Input: part model. Units: mm. Frame: model coordinates. Face numbers are marked on the shaded views. A direction names the side the tool comes from. Give positions to 0.01 mm unless a question says otherwise; leave off trailing zeros. Loops run counter-clockwise (first coordinate to the right, second up) from the corner with the lowest first, then second, coordinate; pieces in that order, holes last. Notation, with made-up numbers: (9, 32.25) - (20, 32.25) arc R3 ccw to (20, 36.25) - close; hole circle Ø1 at (7, -25). An arc over 180 degrees is marked (long way). One line per question, with ' | ' between items. Start each with the question number.
from build123d import *

# Parameters (mm, degrees)
SKETCH_1_R          = 25
SKETCH_1_R_2        = 10
EXTRUDE_1_DEPTH     = 50
EXTRUDE_2_DEPTH     = 12.5
CUT_EXTRUDE_1_DEPTH = 74.993242935
SKETCH_5_R          = 5
CUT_EXTRUDE_2_DEPTH = 124.51619327


with BuildPart() as part:
    # 草图1 → 凸台-拉伸1 (new body)
    with BuildSketch(Plane(origin=(0, 0, 0), x_dir=(1, 0, 0), z_dir=(0, 1, 0))):
        with Locations(Location((0, 0, 0), (0, 0, 270))):
            Circle(SKETCH_1_R)
        with Locations(Location((0, 0, 0), (0, 0, 270))):
            Circle(SKETCH_1_R_2, mode=Mode.SUBTRACT)
    extrude(amount=EXTRUDE_1_DEPTH)

    # 草图2 → 凸台-拉伸2 (add, symmetric)
    with BuildSketch(Plane.XY):
        with BuildLine():
            Line((-25, 50), (25, 50))
            Line((25, 50), (25, 90))
            ThreePointArc((25, 90), (0, 115), (-25, 90))
            Line((-25, 90), (-25, 50))
        make_face()
    extrude(amount=EXTRUDE_2_DEPTH, both=True)

    # 草图4 → 切除-拉伸1 (cut, through all)
    with BuildSketch(Plane.XZ.offset(-50)):
        with BuildLine():
            Line((21.650635095, -12.5), (25, -12.5))
            Line((25, -12.5), (25, 0))
            ThreePointArc((25, 0), (24.148145657, -6.470476128), (21.650635095, -12.5))
        make_face()
        with BuildLine():
            ThreePointArc((21.650635095, 12.5), (24.148145657, 6.470476128), (25, 0))
            Line((25, 0), (25, 12.5))
            Line((25, 12.5), (21.650635095, 12.5))
        make_face()
        with BuildLine():
            Line((-25, 0), (-25, -12.5))
            Line((-25, -12.5), (-21.650635095, -12.5))
            ThreePointArc((-21.650635095, -12.5), (-24.148145657, -6.470476128), (-25, 0))
        make_face()
        with BuildLine():
            Line((-25, 12.5), (-25, 0))
            ThreePointArc((-25, 0), (-24.148145657, 6.470476128), (-21.650635095, 12.5))
            Line((-21.650635095, 12.5), (-25, 12.5))
        make_face()
    extrude(amount=-CUT_EXTRUDE_1_DEPTH, mode=Mode.SUBTRACT)

    # 草图5 → 切除-拉伸2 (cut, through all)
    with BuildSketch(Plane.XY.offset(12.5)):
        with Locations((0, 100)):
            Circle(SKETCH_5_R)
        with Locations((0, 60)):
            Circle(SKETCH_5_R)
    extrude(amount=-CUT_EXTRUDE_2_DEPTH, mode=Mode.SUBTRACT)


solid = part.part
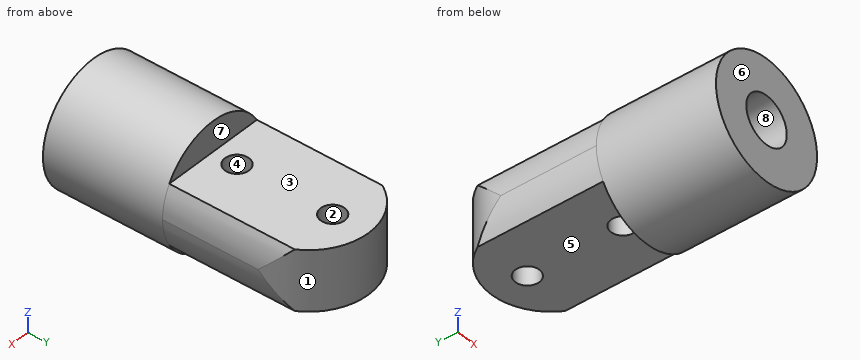
Q1. Section D-D, the plane x = 17. Output: boundary loops of the cut face in (y, z).
Q2. First-contact query: pin 1 (3 mm diameter, centred on x = -5, y = 19, fed in from -Z); pin 2 (4 mm diameter, centred on x = -1, z = 18, fed in from +Y); pin 3 (1.5 mm diameter, centred on x = 15, z = -7, fed in from +Y); pin 4 (8 mm diameter, centred on x = 0, y = 100, fed in from -Z). Flat tips, straight axial feed; report the tip coordinate or a pass-through.
Q3. Section C-C, the plane z = 3. Output: boundary loops of the cut face in (x, y).
Q4. Access query for the marked faces 5, 6, 7 and 8. Directions: +Z, -Z, +X, -X, +Y, -Y. A direction counts if a zero-diameter tool reaches every point of the face in a straight line with its end or side. Return the directions, or none.
Q5. Section B-B, the plane x = 0. Output: boundary loops of the cut face in (y, z).
Q6. Draft query along X for the marked faces 1, 2, 3 and 4. Return one class per face: +X half, -X half, draft (parallel to the pull), parting line (faces both ways), or undercut.
Q7. Line query: L1, parallel to Y at x = 0, z = 7; L2, parallel to X at y = 23.5, z = 0; L3, parallel to Y at x = -1, z = 6.5. Output: solid intervals per line, ascending. Write a range as from..to.
Q8. Section A-A, the plane y = 60. Output: boundary loops of the cut face in (x, z), plus the area to 3 significant figures.
Solved:
1) outline: (0, -18.33) - (50, -18.33) - (50, -12.5) - (108.33, -12.5) - (108.33, 12.5) - (50, 12.5) - (50, 18.33) - (0, 18.33) - close
2) pin 1: stops at z = -24.75 | pin 2: stops at y = 50 | pin 3: stops at y = 110.54 | pin 4: passes through
3) outline: (-24.82, 0) - (-9.54, 0) - (-9.54, 50) - (9.54, 50) - (9.54, 0) - (24.82, 0) - (24.82, 93) arc R25 ccw to (-24.82, 93) - close; hole circle Ø10 at (0, 60); hole circle Ø10 at (0, 100)
4) face 5: -Z, +X, -X, +Y | face 6: +Z, -Z, +X, -X, -Y | face 7: +Z, +X, -X, +Y | face 8: -Y
5) outline: (0, -25) - (50, -25) - (50, -12.5) - (55, -12.5) - (55, 12.5) - (50, 12.5) - (50, 25) - (0, 25) - (0, 10) - (50, 10) - (50, -10) - (0, -10) - close; (65, -12.5) - (95, -12.5) - (95, 12.5) - (65, 12.5) - close; (105, -12.5) - (115, -12.5) - (115, 12.5) - (105, 12.5) - close
6) face 1: parting line | face 2: undercut | face 3: draft | face 4: undercut
7) L1: y = 50..55, 65..95, 105..115 | L2: x = -25..-10, 10..25 | L3: y = 50..55.1, 64.9..95.1, 104.9..114.98
8) outline: (-21.65, -12.5) - (-5, -12.5) - (-5, 12.5) - (-21.65, 12.5) arc R25 ccw to start; (5, -12.5) - (21.65, -12.5) arc R25 ccw to (21.65, 12.5) - (5, 12.5) - close | area: 946 mm²
